The listing builds one solid part. Answer for the finished solid, in the listing's coordinates (mm). A direction names the side the tool comes from. Coordinates: 2 decimals unless noted, no trailing zeros. Loops run counter-clockwise (first coordinate to the right, second up) from the corner with the lowest first, then second, coordinate; pieces in that order, holes last. Notation, with made-up numbers: (22, 18) - (67, 18) arc R18 ccw to (67, 43) - close; hole circle Ø6 at (52, 60). An arc over 180 degrees is marked (long way). Return JSON: item names as keys, results as strings. Group by question number.
1. Section D-D (x = 98.52) is taken. Write down the section's boundary in (y, z), and give its area (3 significant figures).
2. The mould has two halves that part along X. Classify faces 1 (the face through (189, 5, 2)), 2 (the face through (120.5, 18.41, 2.54)), 3 (the face through (76.667, 77, 2)): pulls with the +X half, pulls with the -X half, needs draft (parallel to the pull), parting line crosses it, or undercut.
3. Which of the six approach directions +Z, -Z, +X, -X, +Y, -Y give full straight-line access (tool end or side, diameter ignored) to faces 4 (the face through (225, 64, 2)), 5 (the face through (227, 26.667, 2)), 6 (the face through (25, 20, 3)), 7 (the face through (5, 16, 2))?
4. Each of these flat-tipped pins is pushed along its axis until it touches: P1, Ø1.5, axis at y = 1.5, z = 3.5, coming from the -X side; P2, Ø2.5, axis at y = 20.5, z = 1.5, coming from the -X side. Where does it stop, or does it pass through?
5. Find the intervals of material crossed by line 1 along Y through (x, z) = (30, 3.5); line 2 along X through (y, z) = (43, 4.2); line 3 along X through (y, z) = (55, 0.55), in increasing order.
6. Section A-A (y = 50) is taken. Write down the section's boundary in (x, z).
7. Section B-B (x = 65) is taken. Write down the section's boundary in (y, z), and give its area (4 significant figures).
8. Section C-C (y = 20) is taken. Write down the section's boundary in (x, z).
```python
from build123d import *

# Parameters (mm, degrees)
CROQUIS1_R              = 1.5
CROQUIS1_W              = 44
CROQUIS1_H              = 26
CROQUIS1_W_2            = 5
CROQUIS1_H_2            = 26.666666666
CROQUIS1_W_3            = 76.666666666
CROQUIS1_H_3            = 5
SALIENTE_EXTRUIR1_DEPTH = 5
CROQUIS2_R              = 4.15
CORTAR_EXTRUIR1_DEPTH   = 10
CROQUIS3_W              = 19
CROQUIS3_H              = 13
CORTAR_EXTRUIR2_DEPTH   = 10
CROQUIS4_R              = 4.15
CORTAR_EXTRUIR3_DEPTH   = 10
CROQUIS5_R              = 6
CORTAR_EXTRUIR4_DEPTH   = 10


with BuildPart() as part:
    # Croquis1 → Saliente-Extruir1 (new body)
    with BuildSketch(Plane.XY):
        Polygon((5, 26.666666667), (5, 5), (76.666666667, 5), (153.333333333, 5), (225, 5), (225, 26.666666667), (225, 53.333333333), (225, 75), (153.333333333, 75), (76.666666667, 75), (5, 75), (5, 53.333333333), align=None)
        with Locations((30, 39)):
            Circle(CROQUIS1_R, mode=Mode.SUBTRACT)
        with Locations((83.04, 39)):
            Circle(CROQUIS1_R, mode=Mode.SUBTRACT)
        with Locations((56.52, 52)):
            Rectangle(CROQUIS1_W, CROQUIS1_H, mode=Mode.SUBTRACT)
        with Locations((30, 65)):
            Circle(CROQUIS1_R, mode=Mode.SUBTRACT)
        with Locations((83.04, 65)):
            Circle(CROQUIS1_R, mode=Mode.SUBTRACT)
        with Locations((227.5, 40)):
            Rectangle(CROQUIS1_W_2, CROQUIS1_H_2)
        with Locations((115, 2.5)):
            Rectangle(CROQUIS1_W_3, CROQUIS1_H_3)
        with Locations((2.5, 40)):
            Rectangle(CROQUIS1_W_2, CROQUIS1_H_2)
        with Locations((115, 77.5)):
            Rectangle(CROQUIS1_W_3, CROQUIS1_H_3)
    extrude(amount=SALIENTE_EXTRUIR1_DEPTH)

    # Croquis2 → Cortar-Extruir1 (cut)
    with BuildSketch(Plane.XY.offset(5)):
        with Locations((96.666666667, 20)):
            Circle(CROQUIS2_R)
        with Locations((116.666666667, 20)):
            Circle(CROQUIS2_R)
        with Locations((136.666666667, 20)):
            Circle(CROQUIS2_R)
    extrude(amount=-CORTAR_EXTRUIR1_DEPTH, mode=Mode.SUBTRACT)

    # Croquis3 → Cortar-Extruir2 (cut)
    with BuildSketch(Plane.XY.offset(5)):
        with Locations((34.5, 20.5)):
            Rectangle(CROQUIS3_W, CROQUIS3_H)
    extrude(amount=-CORTAR_EXTRUIR2_DEPTH, mode=Mode.SUBTRACT)

    # Croquis4 → Cortar-Extruir3 (cut)
    with BuildSketch(Plane.XY.offset(5)):
        with Locations((65, 20)):
            Circle(CROQUIS4_R)
        with Locations((80, 20)):
            Circle(CROQUIS4_R)
    extrude(amount=-CORTAR_EXTRUIR3_DEPTH, mode=Mode.SUBTRACT)

    # Croquis5 → Cortar-Extruir4 (cut)
    with BuildSketch(Plane.XY.offset(5)):
        with Locations((98.52, 50)):
            Circle(CROQUIS5_R)
        with Locations((120.52, 50)):
            Circle(CROQUIS5_R)
    extrude(amount=-CORTAR_EXTRUIR4_DEPTH, mode=Mode.SUBTRACT)


solid = part.part
```
The answers:
{
 "1": {"outline": "(0, 0) - (16.29, 0) - (16.29, 5) - (0, 5) - close; (23.71, 0) - (44, 0) - (44, 5) - (23.71, 5) - close; (56, 0) - (80, 0) - (80, 5) - (56, 5) - close", "area": "303 mm2"},
 "2": {"face 1": "needs draft", "face 2": "undercut", "face 3": "pulls with the -X half"},
 "3": {"face 4": "+Z, -Z, +X, +Y", "face 5": "+Z, -Z, +X, -Y", "face 6": "+Z, -Z", "face 7": "+Z, -Z, -X, -Y"},
 "4": {"P1": "stops at x = 76.67", "P2": "stops at x = 5"},
 "5": {"line 1": "y = 5 to 14, 27 to 37.5, 40.5 to 63.5, 66.5 to 75", "line 2": "x = 0 to 34.52, 78.52 to 230", "line 3": "x = 5 to 34.52, 78.52 to 95.2, 101.84 to 117.2, 123.84 to 225"},
 "6": {"outline": "(0, 0) - (34.52, 0) - (34.52, 5) - (0, 5) - close; (78.52, 0) - (92.52, 0) - (92.52, 5) - (78.52, 5) - close; (104.52, 0) - (114.52, 0) - (114.52, 5) - (104.52, 5) - close; (126.52, 0) - (230, 0) - (230, 5) - (126.52, 5) - close"},
 "7": {"outline": "(5, 0) - (15.85, 0) - (15.85, 5) - (5, 5) - close; (24.15, 0) - (39, 0) - (39, 5) - (24.15, 5) - close; (65, 0) - (75, 0) - (75, 5) - (65, 5) - close", "area": "178.5 mm2"},
 "8": {"outline": "(5, 0) - (25, 0) - (25, 5) - (5, 5) - close; (44, 0) - (60.85, 0) - (60.85, 5) - (44, 5) - close; (69.15, 0) - (75.85, 0) - (75.85, 5) - (69.15, 5) - close; (84.15, 0) - (92.52, 0) - (92.52, 5) - (84.15, 5) - close; (100.82, 0) - (112.52, 0) - (112.52, 5) - (100.82, 5) - close; (120.82, 0) - (132.52, 0) - (132.52, 5) - (120.82, 5) - close; (140.82, 0) - (225, 0) - (225, 5) - (140.82, 5) - close"}
}
